The drawing under review shows one solid part. Ordinate dimensions are in mm from its lowest x, y, z. A direction names the side the tool comes from. Coordinates: 2 decimals unless noted, no trailing zeros. Write each loop counter-clockwise with the first axis right and the second up, starting at its lowest first coordinate (ties: lowest second). Pieces come first, ordered by that corner, then holes.
1) We need section B-B on z = 6.5. Write out the cut boundary in (x, y).
2) We need section A-A on y = 6. Write out the cut boundary in (x, z), then the cut area to 3 significant figures.
3) For the marked faces 1, 2, 3 and 4, list the 3-axis set-ups (+Z, -Z, +X, -X, +Y, -Y) from which the entire face can be reached by the end or side of a thin tool; tool diameter is ignored.
4) Insertion check: P1, Ø5, axis at x = 32, z = 15, coming from the +Y side; P2, Ø1.8, axis at x = 31, y = 23, coming from the +Z side; P3, Ø4, axis at x = 16, z = 7.5, coming from the -Y side. Each pin has a flat end and moves straight along its axis. Give the tip position at first contact, or say it passes through.
5) We need section C-C on y = 15. Write out the cut boundary in (x, z).
6) To check wall thickness, follow line 1 along Y through (x, z) = (23.5, 16.5); line 2 along X through (y, z) = (9, 34); line 3 along Y through (x, z) = (31.5, 26). State the ranges of each line that lie inside material, in increasing order.
7) We need section D-D on x = 5. Write out the cut boundary in (y, z), then the cut area to 3 significant figures.
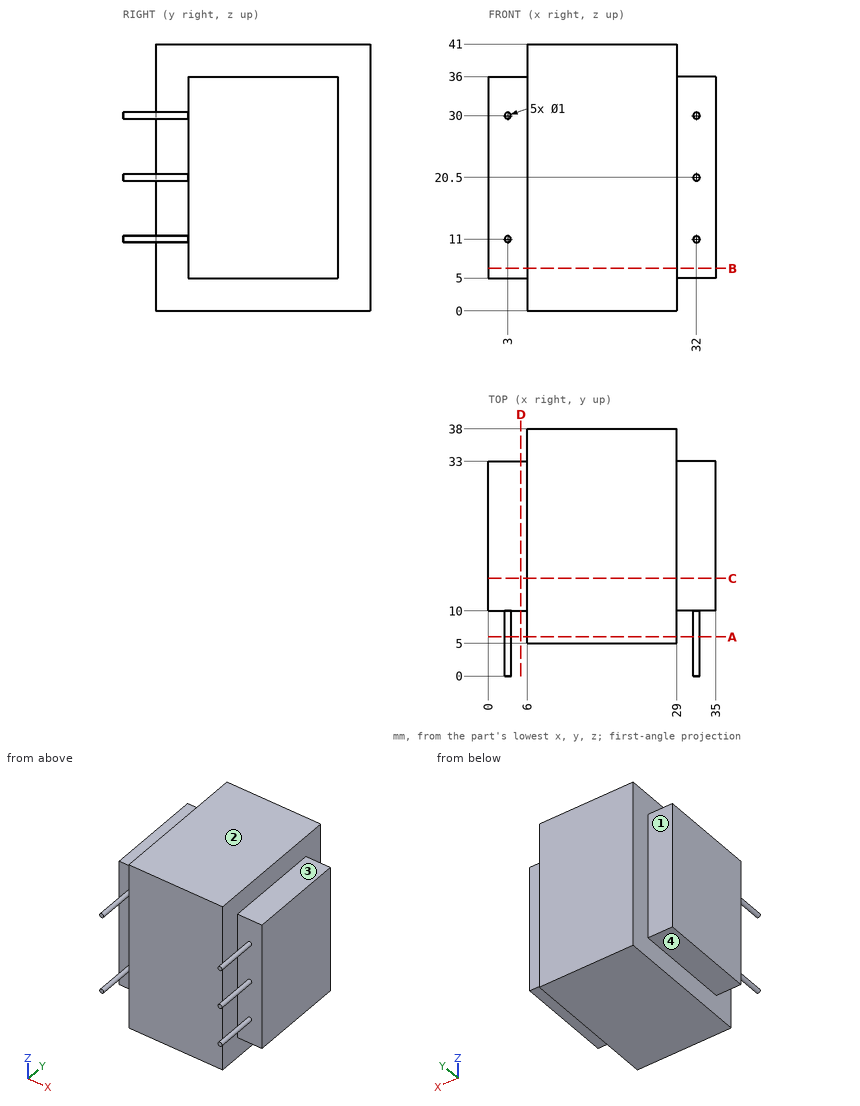
Result:
1. outline: (0, 10) - (6, 10) - (6, 5) - (29, 5) - (29, 10) - (35, 10) - (35, 33) - (29, 33) - (29, 38) - (6, 38) - (6, 33) - (0, 33) - close
2. outline: circle Ø1 at (3, 11); circle Ø1 at (3, 30); (6, 0) - (29, 0) - (29, 41) - (6, 41) - close; circle Ø1 at (32, 11); circle Ø1 at (32, 20.5); circle Ø1 at (32, 30)
2. area: 947 mm2
3. face 1: +Z, -Z, -X, +Y
3. face 2: +Z, +X, -X, +Y, -Y
3. face 3: +Z, +X, +Y, -Y
3. face 4: -Z, -X, +Y, -Y
4. P1: stops at y = 33
4. P2: stops at z = 36
4. P3: stops at y = 5
5. outline: (0, 5) - (6, 5) - (6, 0) - (29, 0) - (29, 5) - (35, 5) - (35, 36) - (29, 36) - (29, 41) - (6, 41) - (6, 36) - (0, 36) - close
6. line 1: y = 5 to 38
6. line 2: x = 6 to 29
6. line 3: y = 10 to 33
7. outline: (10, 5) - (33, 5) - (33, 36) - (10, 36) - close
7. area: 713 mm2
